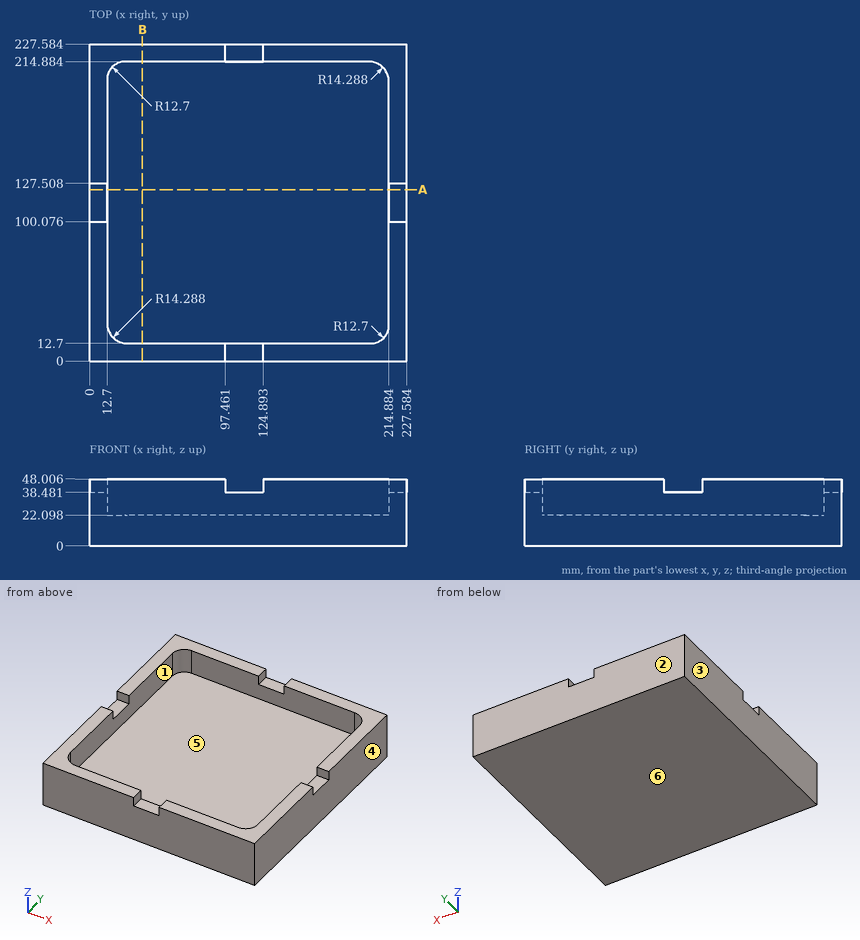
Can you work these out from the drawing? Everything is in mm from the part's minimum corner. A direction names the side the tool comes from. Round coordinates to 2 decimals unless told otherwise and drop trailing zeros. Loops run counter-clockwise (first coordinate to the right, second up) from the corner with the lowest first, then second, coordinate; pieces in that order, holes last.
1. If I drill on line 1 along X through (y, z) = (162, 33.5) (1 decimal); line 2 along Y through (x, z) = (9.5, 40) (1 decimal); line 3 along Z through (x, y) = (147, 189.5), over which ranges is the centre line in solid material (lowest first)?
Answer list:
line 1: x = 0 to 12.7, 214.9 to 227.6
line 2: y = 0 to 100.1, 127.5 to 227.6
line 3: z = 0 to 22.1
2. If we section it at A-A on y = 123: Write out the boundary of the cut face in (x, z) (1 decimal).
Answer list:
outline: (0, 0) - (227.6, 0) - (227.6, 38.5) - (214.9, 38.5) - (214.9, 22.1) - (12.7, 22.1) - (12.7, 38.5) - (0, 38.5) - close
3. If we section it at B-B on x = 38: Write out the boundary of the cut face in (y, z) (1 decimal).
Answer list:
outline: (0, 0) - (227.6, 0) - (227.6, 48) - (214.9, 48) - (214.9, 22.1) - (12.7, 22.1) - (12.7, 48) - (0, 48) - close
4. Which directions (+Z, -Z, +X, -X, +Y, -Y) give clear straight access to the entire face, cutting with the end or side of a thin tool? Please do the marked faces 5 and 6.
Answer list:
face 5: +Z
face 6: -Z, +X, -X, +Y, -Y
5. For P1, Ø10, axis at x = 116, y = 5, coming from the +Z side; P2, Ø6, axis at x = 101, y = 114.5, coming from the +Z side, each with a flat end and sliding along its axis, tell me the tip position at first contact or that it passes through.
Answer list:
P1: stops at z = 38.48
P2: stops at z = 22.1
6. We'd pull the mould along X, two halves only. Please class the marked faces 1, 2, 3 and 4: +X half, -X half, draft (parallel to the pull), parting line (faces both ways), or undercut.
Answer list:
face 1: undercut
face 2: draft
face 3: -X half
face 4: +X half
